Geometry: final body of the model. Coordinates: model frame, mm. A direction names the side the tool comes from. Round coordinates to 2 decimals unless told otherwise and drop trailing zeros. Write each loop counter-clockwise with the first axis right and the second up, starting at its lowest first coordinate (ties: lowest second). Pieces come first, ordered by that corner, then holes. Notation, with made-up numbers: (51.5, 84.5) - (91.5, 84.5) arc R17 ccw to (91.5, 107.5) - close; hole circle Ø6 at (42.5, 24). An arc over 180 degrees is marked (long way). Write each question's results on one line, items separated by ' | '.
from build123d import *

# Parameters (mm, degrees)
SKETCH2_R           = 30
SKETCH2_R_2         = 15
BOSS_EXTRUDE1_DEPTH = 45
SKETCH5_R           = 3.4
CUT_EXTRUDE2_DEPTH  = 15
SKETCH7_R           = 2.5
CUT_EXTRUDE3_DEPTH  = 23
SKETCH8_W           = 8
SKETCH8_H           = 6
CUT_EXTRUDE4_DEPTH  = 62.846584554


with BuildPart() as part:
    # Sketch2 → Boss-Extrude1 (new body)
    with BuildSketch(Plane(origin=(0, 0, 0), x_dir=(1, 0, 0), z_dir=(0, 1, 0))):
        with Locations(Location((0, 0, 0), (0, 0, 90))):
            Circle(SKETCH2_R)
        with Locations(Location((0, 0, 0), (0, 0, 90))):
            Circle(SKETCH2_R_2, mode=Mode.SUBTRACT)
    extrude(amount=BOSS_EXTRUDE1_DEPTH)

    # Sketch5 → Cut-Extrude2 (cut)
    with BuildSketch(Plane(origin=(0, 45, 0), x_dir=(1, 0, 0), z_dir=(0, 1, 0))):
        with Locations(Location((22.5, 0, 0), (0, 0, 270))):
            Circle(SKETCH5_R)
        with Locations(Location((-22.5, 0, 0), (0, 0, 270))):
            Circle(SKETCH5_R)
    extrude(amount=-CUT_EXTRUDE2_DEPTH, mode=Mode.SUBTRACT)

    # Sketch7 → Cut-Extrude3 (cut)
    with BuildSketch(Plane.XY.offset(30)):
        with Locations((0, 35)):
            Circle(SKETCH7_R)
        with Locations((0, 15)):
            Circle(SKETCH7_R)
    extrude(amount=-CUT_EXTRUDE3_DEPTH, mode=Mode.SUBTRACT)

    # Sketch8 → Cut-Extrude4 (cut, through all)
    with BuildSketch(Plane(origin=(0, 45, 0), x_dir=(1, 0, 0), z_dir=(0, 1, 0))):
        with Locations((0, 15.7)):
            Rectangle(SKETCH8_W, SKETCH8_H)
    extrude(amount=-CUT_EXTRUDE4_DEPTH, mode=Mode.SUBTRACT)


solid = part.part
Q1. Section query B-B, the plane z = 0. Return loops of the section in (x, y).
Answer block:
outline: (-30, 0) - (-15, 0) - (-15, 45) - (-19.1, 45) - (-19.1, 30) - (-25.9, 30) - (-25.9, 45) - (-30, 45) - close; (15, 0) - (30, 0) - (30, 45) - (25.9, 45) - (25.9, 30) - (19.1, 30) - (19.1, 45) - (15, 45) - close
Q2. Section query D-D, the plane y = 35. Return loops of the section in (x, z), plus the area to 3 significant figures.
Answer block:
outline: (-4, -18.7) - (-4, -14.46) arc R15 cw to (-2.5, 14.79) - (-2.5, 29.9) arc R30 ccw (long way) to (2.5, 29.9) - (2.5, 14.79) arc R15 cw to (4, -14.46) - (4, -18.7) - close; hole circle Ø6.8 at (-22.5, 0); hole circle Ø6.8 at (22.5, 0) | area: 1,940 mm2
Q3. Ray query, line 1 along X through (y, z) = (41.5, 0); line 2 along Y through (x, z) = (0, 26.75); line 3 along X through (y, z) = (25, 0). Return the intervals inside material, ascending.
Answer block:
line 1: -30 to -25.9, -19.1 to -15, 15 to 19.1, 25.9 to 30 | line 2: 0 to 12.5, 17.5 to 32.5, 37.5 to 45 | line 3: -30 to -15, 15 to 30
Q4. Section query C-C, the plane x = -10. Return loops of the section in (y, z), plus the area to 3 significant figures.
Answer block:
outline: (0, -28.28) - (45, -28.28) - (45, -11.18) - (0, -11.18) - close; (0, 11.18) - (45, 11.18) - (45, 28.28) - (0, 28.28) - close | area: 1,540 mm2
Q5. Pin query (flat end, axial travel): pin 1 (5 mm diameter, centred on y = 28.5, z = -17, fed in from -X); pin 2 (3.5 mm diameter, centred on x = 23.5, z = -0.5, fed in from +Y); pin 3 (18 mm diameter, centred on x = 0, z = 0, fed in from +Y); pin 4 (10 mm diameter, centred on y = 18, z = 23, fed in from -X). Return the tip coordinate at first contact, or that it passes through.
Answer block:
pin 1: x = -26.26 | pin 2: y = 30 | pin 3: through | pin 4: x = -24
Q6. Access query for faces 1 (the flat face through (-14, 45, -6)), 2 (the flat face through (-22, 30, 0)), 3 (the flat face through (4, 23, -17)), 4 (the cylindrical face through (-0.54, 32.56, 22.5)). Directions: +Z, -Z, +X, -X, +Y, -Y. A direction counts if a zero-diameter tool reaches every point of the face in a straight line with its end or side. Return the directions, or none.
Answer block:
face 1: +Z, -Z, +X, -X, +Y | face 2: +Y | face 3: +Y, -Y | face 4: +Z
Q7. Mould query, pull axis X, two halves, no side actions, for faces 5 (the flat face through (-14, 0, -6)), 6 (the flat face through (0, 23, -18.7)), 7 (the cylindrical face through (-1.32, 22.18, 29.97)). Classes: pulls with the +X half, pulls with the -X half, needs draft (parallel to the pull), parting line crosses it, or undercut.
Answer block:
face 5: needs draft | face 6: undercut | face 7: parting line crosses it
Q8. Section query A-A, the plane y = 11. Return loops of the section in (x, z), plus the area to 3 significant figures.
Answer block:
outline: circle Ø60 at (0, 0); hole (-4, -18.7) - (4, -18.7) - (4, -14.46) arc R15 ccw (long way) to (-4, -14.46) - close | area: 2,090 mm2
